from build123d import *

# Parameters (mm, degrees)
SKETCH1_R           = 27.5
BOSS_EXTRUDE1_DEPTH = 20
SKETCH2_R           = 6
BOSS_EXTRUDE2_DEPTH = 105
CHAMFER1_SIZE       = 1
CHAMFER2_SIZE       = 2


with BuildPart() as part:
    # Sketch1 → Boss-Extrude1 (new body)
    with BuildSketch(Plane.XY):
        Circle(SKETCH1_R)
    extrude(amount=BOSS_EXTRUDE1_DEPTH)

    # Sketch2 → Boss-Extrude2 (add)
    with BuildSketch(Plane.XY.offset(20)):
        Circle(SKETCH2_R)
    extrude(amount=BOSS_EXTRUDE2_DEPTH)

    # Chamfer1
    chamfer1_edges = [part.edges().sort_by_distance(p)[0] for p in [
        (-6, 0, 125),
    ]]
    chamfer(chamfer1_edges, length=CHAMFER1_SIZE)

    # Chamfer2
    chamfer2_edges = [part.edges().sort_by_distance(p)[0] for p in [
        (-27.5, 0, 0),
        (-27.5, 0, 20),
    ]]
    chamfer(chamfer2_edges, length=CHAMFER2_SIZE)


solid = part.part
Model file for the job. Use its own axes, mm. Coordinates: 2 decimals unless noted, no trailing zeros. Order: outer loops, then holes, each group sorted by start corner. A loop starts at its lowest first (then second) coordinate and runs counter-clockwise, first axis right, second up. Notation, with made-up numbers: M 44.5,64 L 74.5,64 A9 ccw 74.5,68 Z; hole C 32.25,-8.75 d2. An arc over 180 degrees is marked long. Return JSON: item names as keys, results as strings.
1. Flat gauge pins, fed straight in: pin 1 (1 mm diameter, centred on x = -1, z = 21.5, fed in from +Y); pin 2 (4 mm diameter, centred on y = -15, z = 21, fed in from -X); pin 3 (1.5 mm diameter, centred on x = 7, y = 20, fed in from +Z). Where does each tip first touch, or does it go through?
Ans:
{"pin 1": "y = 5.98", "pin 2": "x = -22.19", "pin 3": "z = 20"}
2. Saw through at A-A (x = 0). Give the cut face in (y, z).
Ans:
{"outline": "M -27.5,2 L -25.5,0 L 25.5,0 L 27.5,2 L 27.5,18 L 25.5,20 L 6,20 L 6,124 L 5,125 L -5,125 L -6,124 L -6,20 L -25.5,20 L -27.5,18 Z"}
3. Pull direction Y, two halves, no side cores. Call faces 1 (the face through (5, -5, 20)), 2 (the face through (-6, 0, 71)): +Y half, -Y half, draft (parallel to the pull), parting line (faces both ways), or undercut.
Ans:
{"face 1": "draft", "face 2": "parting line"}
4. Drill centre lines: probe 1 along Z at (x, y) = (-20, -8); probe 2 along X at (y, z) = (1, 30); probe 3 along X at (y, z) = (-3, 18.5). Where is each one in solid material? Low to high.
Ans:
{"probe 1": "0 to 20", "probe 2": "-5.92 to 5.92", "probe 3": "-26.83 to 26.83"}
5. Saw through at C-C (z = 67.5). Give the cut face in (x, y), and give its area (3 significant figures).
Ans:
{"outline": "C 0,0 d12", "area": "113 mm^2"}
